Source: CAD feature listing. Evaluate the final solid. Frame: model axes, mm. A direction names the side the tool comes from. Round coordinates to 2 decimals unless told otherwise and drop trailing zeros. Loops run counter-clockwise (first coordinate to the right, second up) from the corner with the lowest first, then second, coordinate; pieces in that order, holes last.
Item 1: Section query C-C on z = 21. Return loops of the section in (x, y), then the cut area to 3 significant figures.
Item 2: Section query A-A on z = 16.25. Return loops of the section in (x, y), then the cut area to 3 significant figures.
Item 3: Section query D-D on y = -1.5. Return loops of the section in (x, z), then the cut area to 3 significant figures.
Item 4: First-contact query: P1, Ø8, axis at y = -14, z = 17, coming from the -X side; P2, Ø8, axis at x = -76.01, y = -0.68, coming from the +Z side; P3, Ø1.3, axis at x = -52, z = 14, coming from the -Y side. Flat tips, straight axial feed; report the tip coordinate or a pass-through.
Item 5: Ray query, L1, parallel to X at y = -8, z = 17.5; L2, parallel to Z at x = -69.5, y = -5.5; L3, parallel to Z at x = -62, y = -4.5. Return the intervals inside material, ascending.
Item 6: Access query for faces 4 (the flat face through (-49.591, -6, 16)), 5 (the flat face through (-52, -22.803, 17)), 6 (the flat face through (-53.791, -6, 16)), 7 (the flat face through (-52, 11.197, 17)), 8 (the flat face through (-69.991, -6, 16)). Directions: +Z, -Z, +X, -X, +Y, -Y. A direction counts if a zero-diameter tool reaches every point of the face in a straight line with its end or side. Return the directions, or none.
Item 7: Pull-direction query (X, two-part tool) for faces 1 (the flat face through (-96.991, -6, 5)), 2 (the cylindrical face through (-78.506, -0.573, 5.07)), 3 (the cylindrical face through (-51.721, -5.542, 18.474)); classes: released by +X, released by -X, zero draft, split by the parting line, or undercut.
Item 8: Section query B-B on x = -52.5. Return loops of the section in (y, z).
```python
from build123d import *

# Parameters (mm, degrees)
SKETCH1_W                = 74.4
SKETCH1_H                = 39.6
BOSS_EXTRUDE4_DEPTH      = 10
SKETCH4_W                = 4.2
SKETCH4_H                = 34
BOSS_EXTRUDE7_DEPTH      = 15
CUT_EXTRUDE6_DEPTH       = 60.390731662
CUT_EXTRUDE6_DEPTH_BACK  = 8
CUT_EXTRUDE12_DEPTH      = 57.095802048
CUT_EXTRUDE12_DEPTH_BACK = 15
SKETCH7_R                = 2.5
CUT_EXTRUDE13_DEPTH      = 15


with BuildPart() as part:
    # Sketch1 → Boss-Extrude4 (new body)
    with BuildSketch(Plane.XY):
        with Locations((-59.791289062, -5.802714844)):
            Rectangle(SKETCH1_W, SKETCH1_H)
    extrude(amount=BOSS_EXTRUDE4_DEPTH)

    # Sketch4 → Boss-Extrude7 (add)
    with BuildSketch(Plane.XY.offset(10)):
        with Locations((-67.891289062, -5.802714844)):
            Rectangle(SKETCH4_W, SKETCH4_H)
        Polygon((-49.591289063, 11.197285156), (-53.791289062, 11.197285156), (-53.791289062, -22.802714844), (-49.591289063, -22.802714844), align=None)
    extrude(amount=BOSS_EXTRUDE7_DEPTH)

    # Sketch5 → Cut-Extrude6 (cut, two sides: drawn at the far end of the back side and taken through both)
    with BuildSketch(Plane(origin=(-49.591289063, 0, 0), x_dir=(0, 0, -1), z_dir=(1, 0, 0)).offset(-CUT_EXTRUDE6_DEPTH_BACK)):
        with BuildLine():
            Line((-91.244649925, 84.737426344), (-25, 11.197285156))
            ThreePointArc((-25, 11.197285156), (-18.472201779, -5.802714844), (-25, -22.802714844))
            Line((-25, -22.802714844), (-91.244649925, -96.342856031))
            Line((-91.244649925, -96.342856031), (-289.199250877, -96.342856031))
            Line((-289.199250877, -96.342856031), (-289.199250877, 84.737426344))
            Line((-289.199250877, 84.737426344), (-91.244649925, 84.737426344))
        make_face()
    extrude(amount=CUT_EXTRUDE6_DEPTH + CUT_EXTRUDE6_DEPTH_BACK, mode=Mode.SUBTRACT)

    # Sketch6 → Cut-Extrude12 (cut, two sides: drawn at the far end of the back side and taken through both)
    with BuildSketch(Plane(origin=(-65.791289062, 0, 0), x_dir=(0, 0, -1), z_dir=(1, 0, 0)).offset(-CUT_EXTRUDE12_DEPTH_BACK)):
        with BuildLine():
            Line((-91.244649925, -96.342856031), (-25, -22.802714844))
            ThreePointArc((-25, -22.802714844), (-18.472201779, -5.802714844), (-25, 11.197285156))
            Line((-25, 11.197285156), (-91.244649925, 84.737426344))
            Line((-91.244649925, 84.737426344), (-289.199250877, 84.737426344))
            Line((-289.199250877, 84.737426344), (-289.199250877, -96.342856031))
            Line((-289.199250877, -96.342856031), (-91.244649925, -96.342856031))
        make_face()
    extrude(amount=CUT_EXTRUDE12_DEPTH + CUT_EXTRUDE12_DEPTH_BACK, mode=Mode.SUBTRACT)

    # Sketch7 → Cut-Extrude13 (cut)
    with BuildSketch(Plane.XY.offset(10)):
        with Locations((-42.591289062, -11.682714844)):
            Circle(SKETCH7_R)
        with Locations((-42.591289062, -0.682714844)):
            Circle(SKETCH7_R)
        with Locations((-76.008712531, -0.682714844)):
            Circle(SKETCH7_R)
        with Locations((-76.008712531, -11.682714844)):
            Circle(SKETCH7_R)
    extrude(amount=-CUT_EXTRUDE13_DEPTH, mode=Mode.SUBTRACT)


solid = part.part
```
Data:
1. outline: (-69.99, -22.8) - (-65.79, -22.8) - (-65.79, -16.85) - (-69.99, -16.85) - close; (-69.99, 5.24) - (-65.79, 5.24) - (-65.79, 11.2) - (-69.99, 11.2) - close; (-53.79, -22.8) - (-49.59, -22.8) - (-49.59, -16.85) - (-53.79, -16.85) - close; (-53.79, 5.24) - (-49.59, 5.24) - (-49.59, 11.2) - (-53.79, 11.2) - close
1. area: 100 mm2
2. outline: (-69.99, -22.8) - (-65.79, -22.8) - (-65.79, 11.2) - (-69.99, 11.2) - close; (-53.79, -22.8) - (-49.59, -22.8) - (-49.59, 11.2) - (-53.79, 11.2) - close
2. area: 286 mm2
3. outline: (-96.99, 0) - (-78.37, 0) - (-78.37, 10) - (-96.99, 10) - close; (-73.65, 0) - (-44.95, 0) - (-44.95, 10) - (-49.59, 10) - (-49.59, 18.84) - (-53.79, 18.84) - (-53.79, 10) - (-65.79, 10) - (-65.79, 18.84) - (-69.99, 18.84) - (-69.99, 10) - (-73.65, 10) - close; (-40.23, 0) - (-22.59, 0) - (-22.59, 10) - (-40.23, 10) - close
3. area: 724 mm2
4. P1: stops at x = -69.99
4. P2: stops at z = 10
4. P3: stops at y = -22.8
5. L1: x = -69.99 to -65.79, -53.79 to -49.59
5. L2: z = 0 to 18.47
5. L3: z = 0 to 10
6. face 4: +Z, +X, +Y, -Y
6. face 5: +Z, +X, -X, -Y
6. face 6: +Z, +Y, -Y
6. face 7: +Z, +X, -X, +Y
6. face 8: +Z, -X, +Y, -Y
7. face 1: released by -X
7. face 2: undercut
7. face 3: zero draft
8. outline: (-25.6, 0) - (14, 0) - (14, 10) - (11.2, 10) - (11.2, 25) arc R25.4 cw to (-22.8, 25) - (-22.8, 10) - (-25.6, 10) - close
